from build123d import *

# Parameters (mm, degrees)
EXTRUDE_1_DEPTH     = 120
CUT_EXTRUDE_1_REACH = 12
SKETCH_2_R          = 2.25
CUT_EXTRUDE_2_REACH = 12
SKETCH_3_R          = 2.25


with BuildPart() as part:
    # Эскиз1 → Бобышка-Вытянуть1 (new body)
    with BuildSketch(Plane(origin=(0, 0, 0), x_dir=(0, 0, -1), z_dir=(1, 0, 0))):
        Polygon((0, 0), (0, 10), (2, 10), (2, 2), (10, 2), (10, 0), align=None)
    extrude(amount=EXTRUDE_1_DEPTH)

    # Эскиз2 → Вырез-Вытянуть1 (cut, up to next)
    with BuildSketch(Plane.XY, mode=Mode.PRIVATE) as cut_extrude_1_sk1:
        with Locations((97, 5)):
            Circle(SKETCH_2_R)
    cut_extrude_1_tool1 = extrude(cut_extrude_1_sk1.sketch, amount=-CUT_EXTRUDE_1_REACH, mode=Mode.PRIVATE) & part.part
    add(cut_extrude_1_tool1.solids().sort_by_distance((97, 5, 0))[0], mode=Mode.SUBTRACT)
    # Эскиз2 → Вырез-Вытянуть1 (cut, up to next)
    with BuildSketch(Plane.XY, mode=Mode.PRIVATE) as cut_extrude_1_sk2:
        with Locations((17, 5)):
            Circle(SKETCH_2_R)
    cut_extrude_1_tool2 = extrude(cut_extrude_1_sk2.sketch, amount=-CUT_EXTRUDE_1_REACH, mode=Mode.PRIVATE) & part.part
    add(cut_extrude_1_tool2.solids().sort_by_distance((17, 5, 0))[0], mode=Mode.SUBTRACT)

    # Эскиз3 → Вырез-Вытянуть2 (cut, up to next)
    with BuildSketch(Plane.XZ, mode=Mode.PRIVATE) as cut_extrude_2_sk1:
        with Locations((103, -5)):
            Circle(SKETCH_3_R)
    cut_extrude_2_tool1 = extrude(cut_extrude_2_sk1.sketch, amount=-CUT_EXTRUDE_2_REACH, mode=Mode.PRIVATE) & part.part
    add(cut_extrude_2_tool1.solids().sort_by_distance((103, 0, -5))[0], mode=Mode.SUBTRACT)
    # Эскиз3 → Вырез-Вытянуть2 (cut, up to next)
    with BuildSketch(Plane.XZ, mode=Mode.PRIVATE) as cut_extrude_2_sk2:
        with Locations((23, -5)):
            Circle(SKETCH_3_R)
    cut_extrude_2_tool2 = extrude(cut_extrude_2_sk2.sketch, amount=-CUT_EXTRUDE_2_REACH, mode=Mode.PRIVATE) & part.part
    add(cut_extrude_2_tool2.solids().sort_by_distance((23, 0, -5))[0], mode=Mode.SUBTRACT)


solid = part.part
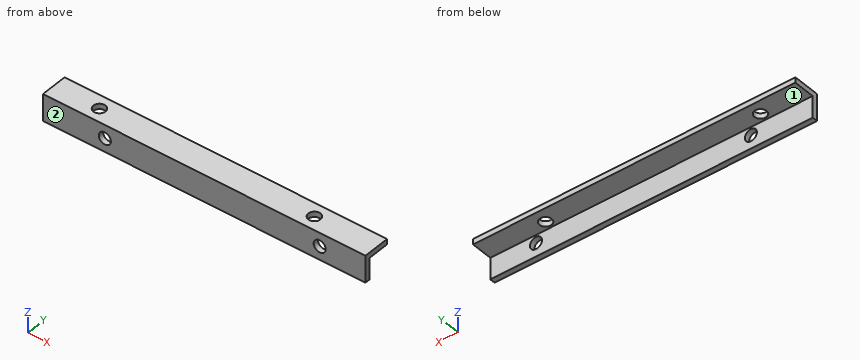
Design review of the part built by this model. Coordinates are the model's own, in mm. Face numbers are marked on the shaded views. A direction names the side the tool comes from. Coordinates: 2 decimals unless noted, no trailing zeros. Order: outer loops, then holes, each group sorted by start corner. A loop starts at its lowest first (then second) coordinate and runs counter-clockwise, first axis right, second up.
Item 1: Take a section at C-C, the plane x = 17. Write out the cut boundary in (y, z), then the cut area to 3 significant figures.
Item 2: For the marked faces 1 and 2, list the 3-axis set-ups (+Z, -Z, +X, -X, +Y, -Y) from which the entire face can be reached by the end or side of a thin tool; tool diameter is ignored.
Item 3: Take a section at A-A, the plane y = 5. Write out the cut boundary in (x, z), then the cut area to 3 significant figures.
Item 4: Take a section at D-D, the plane x = 65. Write out the cut boundary in (y, z).
Item 5: For pin 1 Ø6 at (x, z) = (45.5, -6.5) entering from +Y, flat-tipped, find the tip position at first contact; note if it passes through.
Item 6: Take a section at B-B, the plane z = -5. Write out the cut boundary in (x, y).
Item 7: For line 1 (X direction, y = 1.75, z = -6.25); line 2 (X direction, y = 6.25, z = -1); line 3 (Z direction, x = 103, y = 0.8), list the stretches that pass through material, from the lowest coordinate up.
The answers:
1. outline: (0, -10) - (2, -10) - (2, -2) - (2.75, -2) - (2.75, 0) - (0, 0) - close; (7.25, -2) - (10, -2) - (10, 0) - (7.25, 0) - close
1. area: 27.0 mm2
2. face 1: -Z, +X, -X, +Y
2. face 2: +Z, -Z, +X, -X, -Y
3. outline: (0, -2) - (14.75, -2) - (14.75, 0) - (0, 0) - close; (19.25, -2) - (94.75, -2) - (94.75, 0) - (19.25, 0) - close; (99.25, -2) - (120, -2) - (120, 0) - (99.25, 0) - close
3. area: 222 mm2
4. outline: (0, -10) - (2, -10) - (2, -2) - (10, -2) - (10, 0) - (0, 0) - close
5. pin 1: stops at y = 2
6. outline: (0, 0) - (20.75, 0) - (20.75, 2) - (0, 2) - close; (25.25, 0) - (100.75, 0) - (100.75, 2) - (25.25, 2) - close; (105.25, 0) - (120, 0) - (120, 2) - (105.25, 2) - close
7. line 1: x = 0 to 21.13, 24.87 to 101.13, 104.87 to 120
7. line 2: x = 0 to 15.13, 18.87 to 95.13, 98.87 to 120
7. line 3: z = -10 to -7.25, -2.75 to 0
